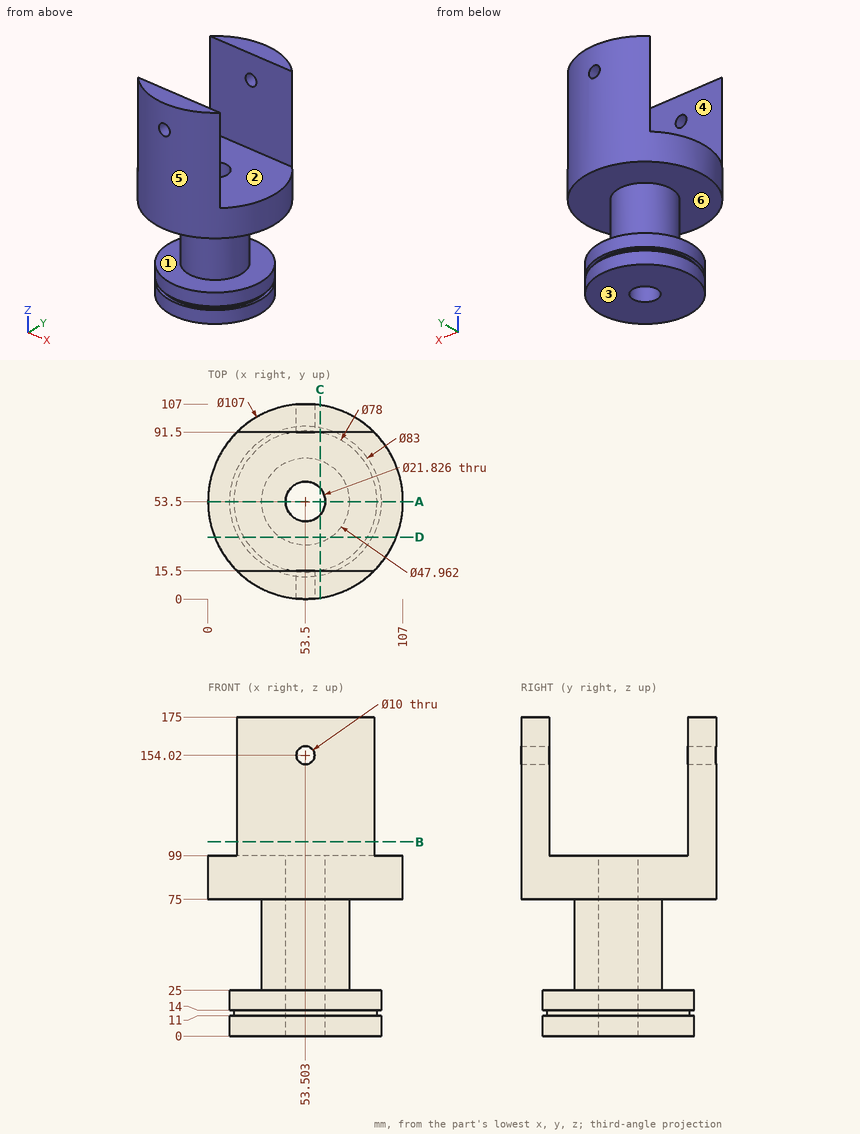
Job drawing, mm, ordinate dimensions from the low corner. One solid piece. A direction names the side the tool comes from. Coordinates: 2 decimals unless noted, no trailing zeros. Write each loop counter-clockwise with the first axis right and the second up, starting at its lowest first coordinate (ties: lowest second). Pieces come first, ordered by that corner, then holes.
Item 1: Probe line 1 (Y direction, x = 54, z = 140.5); line 2 (Z direction, x = 61, y = 78); line 3 (Y direction, x = 53.5, z = 36.5). List the from-to ranges inside material, lowest first.
Item 2: Slice it at B-B (z = 106.5). Write the cut outline in (x, y).
Item 3: Slice it at C-C (x = 61.5). Write the cut outline in (y, z).
Item 4: Mould opens along Y. For the marked faces 4, 5 and 6 say: released by +Y, released by -Y, zero draft, split by the parting line, or undercut.
Item 5: Pin check, flat tips, straight feed: pin 1 (4 mm diameter, centred on x = 67, z = 70.5, fed in from -Y); pin 2 (8 mm diameter, centred on x = 61, y = 67.5, fed in from +Z); pin 3 (10 mm diameter, centred on y = 68, z = 79, fed in from +X); pin 4 (13 mm diameter, centred on x = 53.5, y = 53.5, fed in from -Z). Stop position of each tip, or through.
Item 6: Which spindle directions (+Z, -Z, +X, -X, +Y, -Y) get a long thin tool onto all of the face, cutting with end or side? Do the marked faces 1, 2 and 3. Say none if no direction does.
Item 7: Slice it at D-D (y = 34). Write the cut outline in (x, z) (1 decimal).
Item 8: Slice it at A-A (y = 53.5). Write the cut outline in (x, z).
Results found:
1. line 1: y = 0 to 15.5, 91.5 to 107
1. line 2: z = 0 to 25, 75 to 99
1. line 3: y = 29.52 to 42.59, 64.41 to 77.48
2. outline: (15.84, 15.5) arc R53.5 ccw to (91.16, 15.5) - close; (15.84, 91.5) - (91.16, 91.5) arc R53.5 ccw to start
3. outline: (0.6, 75) - (30.89, 75) - (30.89, 25) - (12.78, 25) - (12.78, 14) - (15.33, 14) - (15.33, 11) - (12.78, 11) - (12.78, 0) - (46.08, 0) - (46.08, 99) - (15.5, 99) - (15.5, 175) - (0.6, 175) - close; (60.92, 0) - (94.22, 0) - (94.22, 11) - (91.67, 11) - (91.67, 14) - (94.22, 14) - (94.22, 25) - (76.11, 25) - (76.11, 75) - (106.4, 75) - (106.4, 175) - (91.5, 175) - (91.5, 99) - (60.92, 99) - close
4. face 4: undercut
4. face 5: split by the parting line
4. face 6: zero draft
5. pin 1: stops at y = 32.46
5. pin 2: stops at z = 99
5. pin 3: stops at x = 106.15
5. pin 4: passes through
6. face 1: none
6. face 2: +Z, +X, -X
6. face 3: -Z, +X, -X, +Y, -Y
7. outline: (3.7, 75) - (39.5, 75) - (39.5, 25) - (16.9, 25) - (16.9, 14) - (19.7, 14) - (19.7, 11) - (16.9, 11) - (16.9, 0) - (90.1, 0) - (90.1, 11) - (87.3, 11) - (87.3, 14) - (90.1, 14) - (90.1, 25) - (67.5, 25) - (67.5, 75) - (103.3, 75) - (103.3, 99) - (3.7, 99) - close
8. outline: (0, 75) - (29.52, 75) - (29.52, 25) - (12, 25) - (12, 14) - (14.5, 14) - (14.5, 11) - (12, 11) - (12, 0) - (42.59, 0) - (42.59, 99) - (0, 99) - close; (64.41, 0) - (95, 0) - (95, 11) - (92.5, 11) - (92.5, 14) - (95, 14) - (95, 25) - (77.48, 25) - (77.48, 75) - (107, 75) - (107, 99) - (64.41, 99) - close
